Autodesk Inventor part; units mm, degrees
ref_plane "YZ Plane" through (0, 0, 0) normal (1, 0, 0) x (0, 1, 0)
ref_plane "XZ Plane" through (0, 0, 0) normal (0, 1, 0) x (-1, 0, 0)
ref_plane "XY Plane" through (0, 0, 0) normal (0, 0, 1) x (1, 0, 0)
sketch "Sketch1" plane through (0, 0, 0) normal (0, 1, 0) x (-1, 0, 0)
  line L0 (0, 0) -> (84, 0)
  line L1 (84, 0) -> (84, -156)
  line L2 (84, -156) -> (0, -156)
  line L3 (0, -156) -> (0, 0)
  line L4 (84, 0) -> (84, -3)
  line L5 (84, -3) -> (81, -3) construction
  line L6 (0, -156) -> (0, -153)
  line L7 (0, -153) -> (3, -153) construction
  line L8 (81, -3) -> (3, -3)
  line L9 (3, -3) -> (3, -153)
  line L10 (3, -153) -> (81, -153)
  line L11 (81, -153) -> (81, -3)
  dimension "d0" = 84
  dimension "d1" = 156
  dimension "d2" = 3
  dimension "d3" = 3
  dimension "d4" = 3
  dimension "d5" = 3
extrude "Extrusion1" add sketch "Sketch1" along normal blind 15 contours L0 L1 L2 L3 | L11 L10 L9 L8
sketch "Sketch2" plane through (0, 15, 0) normal (0, 1, 0) x (1, 0, 0)
  line L0 (-84, 156) -> (-84, 0)
  line L1 (-84, 0) -> (-84, 3)
  line L2 (-84, 3) -> (-81, 3) construction
  line L3 (0, 0) -> (0, 156)
  line L4 (0, 156) -> (0, 153)
  line L5 (0, 153) -> (-3, 153) construction
  line L6 (-81, 3) -> (-3, 3)
  line L7 (-3, 3) -> (-3, 153)
  line L8 (-3, 153) -> (-81, 153)
  line L9 (-81, 153) -> (-81, 3)
  dimension "d8" = 3
  dimension "d9" = 3
  dimension "d10" = 3
  dimension "d11" = 3
extrude "Extrusion2" cut sketch "Sketch2" against normal blind 12
sketch "Sketch5" plane through (0, 0, 0) normal (1, 0, 0) x (0, 0, -1)
  line L0 (0, 15) -> (156, 15)
  line L1 (0, 15) -> (0, 0)
  line L2 (156, 0) -> (0, 0)
  line L3 (0, 0) -> (156, 0)
  line L4 (156, 0) -> (156, 15)
  line L5 (156, 15) -> (153, 15)
  line L6 (3, 3) -> (153, 3)
  line L7 (153, 15) -> (153, 3)
  line L8 (153, 3) -> (83, 3)
  line L9 (83, 3) -> (83, 15)
  line L10 (0, 15) -> (3, 15)
  line L11 (3, 15) -> (3, 3)
  line L12 (3, 15) -> (3, 3)
  line L13 (3, 3) -> (73, 3)
  line L14 (73, 3) -> (73, 15)
  line L15 (83, 15) -> (73, 15)
  dimension "d18" = 3
  dimension "d19" = 12
  dimension "d20" = 70
  dimension "d21" = 70
extrude "Extrusion3" add sketch "Sketch5" along normal blind 27 contours L0 L11 L6 L7 L4 L2 L1 | L0 L9 L6 L14
sketch "Sketch6" plane through (27, 0, 0) normal (1, 0, 0) x (0, 0, -1)
  line L0 (0, 15) -> (0, 0)
  line L1 (156, 0) -> (156, 15)
  line L2 (0, 0) -> (156, 0)
  line L3 (156, 0) -> (156, 15)
  line L4 (156, 15) -> (0, 15)
  line L5 (0, 15) -> (0, 0)
extrude "Extrusion4" add sketch "Sketch6" along normal blind 3
sketch "Sketch8" plane through (-84, 0, -156) normal (-1, 0, 0) x (0, 0, 1)
  line L0 (3, 15) -> (3, 3)
  line L1 (3, 15) -> (3, 3)
  line L2 (3, 3) -> (73, 3)
  line L3 (73, 3) -> (73, 15)
  line L4 (156, 15) -> (153, 15)
  line L5 (153, 15) -> (153, 3)
  line L6 (153, 3) -> (83, 3)
  line L7 (83, 3) -> (83, 15)
  line L8 (83, 15) -> (73, 15)
  line L9 (156, 0) -> (156, 15)
  line L10 (156, 15) -> (156, 0)
  line L11 (156, 0) -> (0, 0)
  line L12 (0, 0) -> (0, 15)
  line L13 (0, 0) -> (0, 15)
  line L14 (0, 15) -> (3, 15)
  dimension "d35" = 70
  dimension "d38" = 12
  dimension "d39" = 70
extrude "Extrusion5" add sketch "Sketch8" along normal blind 27
sketch "Sketch9" plane through (-111, 0, -156) normal (-1, 0, 0) x (0, 0, 1)
  line L0 (0, 0) -> (156, 0)
  line L1 (156, 15) -> (156, 0)
  line L2 (0, 0) -> (156, 0)
  line L3 (156, 0) -> (156, 15)
  line L4 (156, 15) -> (0, 15)
  line L5 (0, 15) -> (0, 0)
extrude "Extrusion6" add sketch "Sketch9" along normal blind 3
sketch "Sketch10" plane through (0, 15, 0) normal (0, 1, 0) x (1, 0, 0)
  line L0 (-3, 3) -> (-81, 3)
  line L1 (-3, 3) -> (-3, 0)
  line L2 (30, 0) -> (-114, 0)
  line L3 (30, 156) -> (30, 0)
  line L4 (30, 156) -> (-3, 156)
  line L5 (-3, 156) -> (-3, 0)
  line L6 (-3, 0) -> (30, 0)
  line L7 (30, 0) -> (30, 156)
  line L8 (-81, 3) -> (-81, 0)
  line L9 (-114, 156) -> (30, 156)
  line L10 (-114, 156) -> (-81, 156)
  line L11 (-81, 156) -> (-81, 0)
  line L12 (-81, 0) -> (-114, 0)
  line L13 (-114, 0) -> (-114, 156)
  line L14 (27, 153) -> (27, 83)
  line L15 (0, 83) -> (0, 153)
  line L16 (27, 153) -> (0, 153)
  line L17 (0, 153) -> (0, 83)
  line L18 (0, 83) -> (27, 83)
  line L19 (27, 83) -> (27, 153)
  line L20 (0, 73) -> (27, 73)
  line L21 (0, 3) -> (27, 3)
  line L22 (27, 73) -> (0, 73)
  line L23 (0, 73) -> (0, 3)
  line L24 (0, 3) -> (27, 3)
  line L25 (27, 3) -> (27, 73)
  line L26 (-84, 153) -> (-84, 83)
  line L27 (-84, 83) -> (-111, 83)
  line L28 (-84, 153) -> (-111, 153)
  line L29 (-111, 153) -> (-111, 83)
  line L30 (-111, 83) -> (-84, 83)
  line L31 (-84, 83) -> (-84, 153)
  line L32 (-84, 73) -> (-84, 3)
  line L33 (-84, 3) -> (-111, 3)
  line L34 (-84, 73) -> (-111, 73)
  line L35 (-111, 73) -> (-111, 3)
  line L36 (-111, 3) -> (-84, 3)
  line L37 (-84, 3) -> (-84, 73)
  point P0 (0, 0)
extrude "Extrusion7" add sketch "Sketch10" along normal blind 10 contours L5 L4 L3 L2 L1 | L8 L2 L13 L9 L11
sketch "Sketch11" plane through (-114, 0, -156) normal (-1, 0, 0) x (0, 0, 1)
  line L0 (0, 25) -> (16, 25)
  line L1 (16, 25) -> (16, 13.8)
  circle A0 centre (16, 13.8) radius 3
  line L2 (156, 15) -> (156, 25)
  line L3 (156, 25) -> (140, 25)
  line L4 (140, 25) -> (140, 13.8)
  circle A1 centre (140, 13.8) radius 3
  dimension "d117" = 16
  dimension "d118" = 11.2
  dimension "d119" = 6
  dimension "d120" = 16
  dimension "d121" = 11.2
  dimension "d122" = 6
extrude "Extrusion8" cut sketch "Sketch11" against normal blind 32
sketch "Sketch12" plane through (30, 0, 0) normal (1, 0, 0) x (0, 0, -1)
  line L0 (0, 25) -> (16, 25)
  line L1 (0, 25) -> (16, 25) construction
  line L2 (16, 25) -> (16, 13.8)
  circle A0 centre (16, 13.8) radius 3
  line L3 (156, 25) -> (140, 25)
  line L4 (140, 25) -> (140, 13.8)
  circle A1 centre (140, 13.8) radius 3
  dimension "d98" = 16
  dimension "d99" = 0
  dimension "d100" = 11.2
  dimension "d101" = 6
  dimension "d102" = 16
  dimension "d103" = 11.2
  dimension "d104" = 6
extrude "Extrusion9" cut sketch "Sketch12" against normal blind 32
sketch "Sketch13" plane through (0, 3, -3) normal (1, 0, 0) x (0, 0, -1)
  line L0 (0, 22) -> (70, 22)
  line L1 (0, 22) -> (55, 22)
  line L2 (55, 22) -> (54.9973, 12)
  circle A0 centre (54.9973, 12) radius 2.5
  line L3 (80, 22) -> (95, 22)
  line L4 (80, 22) -> (150, 22)
  line L5 (95, 22) -> (95, 12)
  circle A1 centre (95, 12) radius 2.5
  point P0 (-3, -3)
  dimension "d105" = 55
  dimension "d106" = 10
  dimension "d107" = 5
  dimension "d108" = 15
  dimension "d109" = 10
  dimension "d110" = 5
sketch "Sketch14" plane through (-84, 3, -153) normal (-1, 0, 0) x (0, 0, 1)
  line L0 (70, 0) -> (70, 22)
  line L1 (70, 22) -> (55, 22)
  line L2 (55, 22) -> (55, 12)
  circle A0 centre (55, 12) radius 2.5
  line L3 (80, 22) -> (95, 22)
  line L4 (95, 22) -> (95, 12)
  circle A1 centre (95, 12) radius 2.5
  point P0 (153, -3)
  point P1 (0, 22)
  point P2 (150, 22)
  dimension "d111" = 15
  dimension "d112" = 10
  dimension "d113" = 5
  dimension "d114" = 15
  dimension "d115" = 10
  dimension "d116" = 5
extrude "Extrusion10" cut sketch "Sketch14" against normal blind 10
extrude "Extrusion11" cut sketch "Sketch13" against normal blind 10
sketch "Sketch15" plane through (-81, 3, -3) normal (1, 0, 0) x (0, 0, -1)
  line L0 (-3, 22) -> (87.2546, 33.7556)
  line L1 (87.2546, 33.7556) -> (153, 12)
  line L2 (-3, 22) -> (-3, 12)
  line L3 (153, 12) -> (150, 12)
  line L4 (153, 12) -> (-3, 12)
extrude "Extrusion12" add sketch "Sketch15" along normal up to surface (78 mm away)
properties part number "prototype 1"
The model under review builds one solid part; all positions refer to its coordinate system, in mm. A direction names the side the tool comes from. Give positions to 0.01 mm unless a question says otherwise; leave off trailing zeros. Write each loop counter-clockwise with the first axis right and the second up, starting at its lowest first coordinate (ties: lowest second). Pieces come first, ordered by that corner, then holes. Notation, with made-up numbers: (-39, 9) - (-19, 9) arc R21 cw to (-19, 48) - close; hole circle Ø3 at (54.5, 11). An arc over 180 degrees is marked (long way). Answer in a Markdown table with one row per item. Add a question column.
1. Insertion check: P1, Ø12, axis at x = -63.5, z = -113.5, coming from the +Y side; P2, Ø5, axis at y = 13.8, z = -16, coming from the -X side; P3, Ø13.5, axis at x = 15.5, z = -25, coming from the +Y side; P4, Ø7, axis at y = 13.8, z = -140, coming from the +X side. Each pin has a flat end and moves straight along its axis. Give the tip position at first contact, or say it passes through.
2. Draft analysis for pull direction Z (two halves, no side actions). For faces 6 (the cylindrical face through (-83.014, 16.774, -16.391)), 7 (the flat face through (-111, 14, -38)), 8 (the flat face through (-81, 30, -76)), state which applies: +Z half, -Z half, draft (parallel to the pull), parting line (faces both ways), or undercut.
3. We need section A-A on z = -85. Write out the cut boundary in (x, y), then the cut area to 3 significant figures.
4. Tool access review of faces 1 (the flat face through (-114, 13, -79)), 2 (the cylindrical face through (28.52, 14.7, -142.86)), 3 (the flat face through (-41, 9, -153)), 4 (the flat face through (-97, 3, -38)), 5 (the cylindrical face through (-83.01, 14.7, -137.14)): name each direction out of +Z, -Z, +X, -X, +Y, -Y from which nothing blocks a thin tool from reaching the whole face with its end or side.
5. We need section D-D on z = -58. Write out the cut boundary in (x, y).
6. Wall thickness on line 1 along X through (y, z) = (23.5, -93); line 2 along X through (y, z) = (9, -19.5); line 3 along Z through (x, y) = (27.8, 13.8): over which ranges is each line inside the solid? List them lowest first. Write a range as [from, to].
7. We need section B-B on y = 21. Write out the cut boundary in (x, z).
8. We need section C-C on z = -140. State how many separate pieces and enclosed holes the cut face has, then the cut area to 3 significant figures.
Ans:
| question | item | result |
|---|---|---|
| 1 | P1 | stops at y = 31.05 |
| 1 | P2 | stops at x = -82 |
| 1 | P3 | stops at y = 3 |
| 1 | P4 | stops at x = 30 |
| 2 | face 6 | undercut |
| 2 | face 7 | undercut |
| 2 | face 8 | draft |
| 3 | outline | (-114, 0) - (30, 0) - (30, 25) - (27, 25) - (27, 3) - (0, 3) - (0, 25) - (-3, 25) - (-3, 36.07) - (-81, 36.07) - (-81, 25) - (-84, 25) - (-84, 3) - (-111, 3) - (-111, 25) - (-114, 25) - close; hole (-81, 3) - (-3, 3) - (-3, 15) - (-81, 15) - close |
| 3 | area | 2,340 mm^2 |
| 4 | face 1 | +Z, -Z, -X, +Y, -Y |
| 4 | face 2 | +X |
| 4 | face 3 | none |
| 4 | face 4 | +Y |
| 4 | face 5 | -X |
| 5 | outline | (-114, 0) - (30, 0) - (30, 25) - (27, 25) - (27, 3) - (0, 3) - (0, 12.5) - (-3, 12.5) - (-3, 3) - (-81, 3) - (-81, 12.5) - (-84, 12.5) - (-84, 3) - (-111, 3) - (-111, 25) - (-114, 25) - close; (-84, 17.5) - (-81, 17.5) - (-81, 15) - (-3, 15) - (-3, 17.5) - (0, 17.5) - (0, 25) - (-3, 25) - (-3, 32.55) - (-81, 32.55) - (-81, 25) - (-84, 25) - close |
| 6 | line 1 | x = [-114, -111], [-84, 0], [27, 30] |
| 6 | line 2 | x = [-114, -111], [-84, -81], [-3, 0], [27, 30] |
| 6 | line 3 | z = [-156, -143], [-137, -19], [-13, 0] |
| 7 | outline | (-114, -156) - (-81, -156) - (-81, -137.87) - (-3, -137.87) - (-3, -156) - (30, -156) - (30, 0) - (-114, 0) - close; hole (-111, -153) - (-84, -153) - (-84, -83) - (-111, -83) - close; hole (-111, -73) - (-84, -73) - (-84, -3) - (-111, -3) - close; hole (0, -153) - (27, -153) - (27, -83) - (0, -83) - close; hole (0, -73) - (27, -73) - (27, -3) - (0, -3) - close |
| 8 | separate pieces | 3 |
| 8 | enclosed holes | 1 |
| 8 | area | 1,050 mm^2 |
